Here's how the part is built. I have some questions about the finished solid (model axes, mm). Face numbers are marked on the shaded views. A direction names the side the tool comes from. Give positions to 0.01 mm unless a question says otherwise; leave off trailing zeros. Loops run counter-clockwise (first coordinate to the right, second up) from the corner with the lowest first, then second, coordinate; pieces in that order, holes last. Notation, with made-up numbers: (72.5, 29) - (78.5, 29) arc R18 ccw to (78.5, 52) - close; hole circle Ø7 at (-14.5, -2.5). An arc over 180 degrees is marked (long way). Use a Markdown table: item, result.
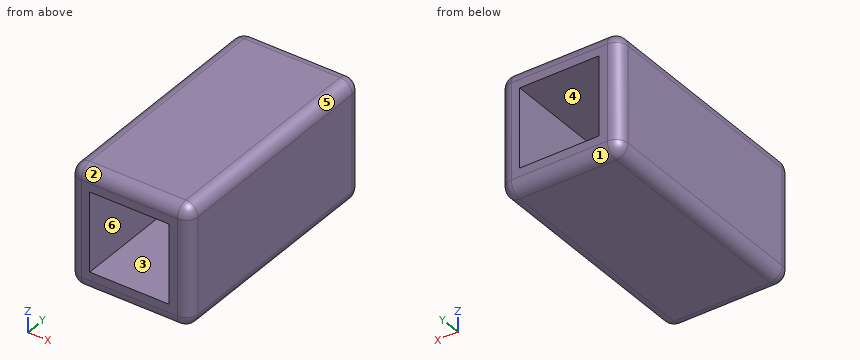
from build123d import *

# Parameters (mm, degrees)
F0_W     = 20
F0_H     = 20
F1_DEPTH = 40
F2_W     = 13.2
F2_H     = 13.2
F3_DEPTH = 18
F4_W     = 13.2
F4_H     = 13.2
F5_DEPTH = 18
F6_R     = 2


with BuildPart() as f1:
    # F0 (on Front) → F1 (new body)
    with BuildSketch(Plane.XZ):
        with Locations((10, 10)):
            Rectangle(F0_W, F0_H)
    extrude(amount=F1_DEPTH)

    # F2 (on face) → F3 (cut)
    with BuildSketch(Plane(origin=(0, 0, 0), x_dir=(-1, 0, 0), z_dir=(0, 1, 0))):
        with Locations((-10, 10)):
            Rectangle(F2_W, F2_H)
    extrude(amount=-F3_DEPTH, mode=Mode.SUBTRACT)

    # F4 (on face) → F5 (cut)
    with BuildSketch(Plane.XZ.offset(40)):
        with Locations((10, 10)):
            Rectangle(F4_W, F4_H)
    extrude(amount=-F5_DEPTH, mode=Mode.SUBTRACT)

    # F6
    f6_edges = [f1.edges().sort_by_distance(p)[0] for p in [
        (0, -20, 0),
        (20, -20, 0),
        (10, 0, 0),
        (10, -40, 0),
        (0, -20, 20),
        (0, 0, 10),
        (0, -40, 10),
        (20, -20, 20),
        (10, 0, 20),
        (10, -40, 20),
        (20, 0, 10),
        (20, -40, 10),
    ]]
    fillet(f6_edges, radius=F6_R)


solid = f1.part
(1) Will this pin go through, and if not, where does the flat tip stop? pin 1 (6.5 mm diameter, centred on x = 7, z = 10.5, fed in from -Y).
A:
| item | result |
|---|---|
| pin 1 | y = -22 |
(2) Suppose I cut it at C-C on x = 12.75. Write out the boundary of the cut face in (y, z), plus the area to 3 significant figures.
A:
| item | result |
|---|---|
| outline | (-40, 2) arc R2 ccw to (-38, 0) - (-2, 0) arc R2 ccw to (0, 2) - (0, 3.4) - (-18, 3.4) - (-18, 16.6) - (0, 16.6) - (0, 18) arc R2 ccw to (-2, 20) - (-38, 20) arc R2 ccw to (-40, 18) - (-40, 16.6) - (-22, 16.6) - (-22, 3.4) - (-40, 3.4) - close |
| area | 321 mm2 |
(3) We'd pull the mould along Z, two halves only. Please class the marked faces 1, 2 and 3: pulls with the +Z half, pulls with the -Z half, needs draft (parallel to the pull), parting line crosses it, or undercut.
A:
| item | result |
|---|---|
| face 1 | pulls with the -Z half |
| face 2 | pulls with the +Z half |
| face 3 | undercut |
(4) Suppose I cut it at A-A on z = 11. Write out the boundary of the cut face in (x, y).
A:
| item | result |
|---|---|
| outline | (0, -38) arc R2 ccw to (2, -40) - (3.4, -40) - (3.4, -22) - (16.6, -22) - (16.6, -40) - (18, -40) arc R2 ccw to (20, -38) - (20, -2) arc R2 ccw to (18, 0) - (16.6, 0) - (16.6, -18) - (3.4, -18) - (3.4, 0) - (2, 0) arc R2 ccw to (0, -2) - close |
(5) On a 3-axis mill with a long thin cutter (end or side, diameter ignored), from which of +Z, -Z, +X, -X, +Y, -Y can I reach the whole of each face in a straight line? I mean the marked faces 4, 5 and 6. Say none if no direction works.
A:
| item | result |
|---|---|
| face 4 | +Y |
| face 5 | +Z, +X, +Y, -Y |
| face 6 | -Y |
(6) Suppose I cut it at B-B on y = -13. Write out the boundary of the cut face in (x, z), plus the area to 3 significant figures.
A:
| item | result |
|---|---|
| outline | (0, 2) arc R2 ccw to (2, 0) - (18, 0) arc R2 ccw to (20, 2) - (20, 18) arc R2 ccw to (18, 20) - (2, 20) arc R2 ccw to (0, 18) - close; hole (3.4, 3.4) - (16.6, 3.4) - (16.6, 16.6) - (3.4, 16.6) - close |
| area | 222 mm2 |
(7) If I drill on line 1 (Z direction, x = 4, y = -27.5); line 2 (Y direction, x = 4.25, z = 4), over which ranges is the centre line in solid material (lowest first)?
A:
| item | result |
|---|---|
| line 1 | 0 to 3.4, 16.6 to 20 |
| line 2 | -22 to -18 |
